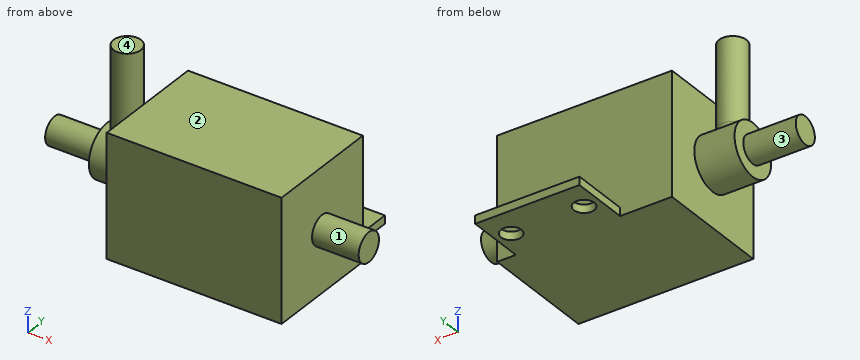
from build123d import *

# Parameters (mm, degrees)
SKETCH1_W                            = 30
SKETCH1_H                            = 20
BOSS_EXTRUDE1_DEPTH                  = 21
SKETCH2_W                            = 17.9
SKETCH2_H                            = 1.4
BOSS_EXTRUDE2_DEPTH                  = 10
SKETCH3_R                            = 2.5
BOSS_EXTRUDE3_DEPTH                  = 8
SKETCH4_R                            = 4.5
BOSS_EXTRUDE4_DEPTH                  = 6.9
SKETCH5_R                            = 2.35
BOSS_EXTRUDE5_DEPTH                  = 9
SKETCH7_R                            = 2.35
BOSS_EXTRUDE6_DEPTH                  = 14.2
BOSS_EXTRUDE6_DIRECTION_2_REACH      = 53.391
BOSS_EXTRUDE6_DIRECTION_2_END_RADIUS = 4.5
SKETCH8_2_R                          = 1.75
CUT_EXTRUDE1_DEPTH                   = 56.828666472
SKETCH8_R                            = 1.75
BOSS_EXTRUDE7_DEPTH                  = 27.8


with BuildPart() as part:
    # Sketch1 → Boss-Extrude1 (new body)
    with BuildSketch(Plane.XY):
        with Locations((15, 10)):
            Rectangle(SKETCH1_W, SKETCH1_H)
    extrude(amount=BOSS_EXTRUDE1_DEPTH)

    # Sketch2 → Boss-Extrude2 (add)
    with BuildSketch(Plane(origin=(0, 20, 0), x_dir=(1, 0, 0), z_dir=(0, 1, 0))):
        with Locations((17.85, -0.7)):
            Rectangle(SKETCH2_W, SKETCH2_H)
    extrude(amount=BOSS_EXTRUDE2_DEPTH)

    # Sketch3 → Boss-Extrude3 (add)
    with BuildSketch(Plane(origin=(30, 0, 0), x_dir=(0, 0, -1), z_dir=(1, 0, 0))):
        with Locations((-10.5, 10)):
            Circle(SKETCH3_R)
    extrude(amount=BOSS_EXTRUDE3_DEPTH)

    # Sketch4 → Boss-Extrude4 (add)
    with BuildSketch(Plane.ZY):
        with Locations(Location((10.5, 10, 0), (0, 0, 180))):
            Circle(SKETCH4_R)
    extrude(amount=BOSS_EXTRUDE4_DEPTH)

    # Sketch5 → Boss-Extrude5 (add)
    with BuildSketch(Plane.ZY.offset(6.9)):
        with Locations((10.5, 10)):
            Circle(SKETCH5_R)
    extrude(amount=BOSS_EXTRUDE5_DEPTH)

    # Sketch7 → Boss-Extrude6 (add)
    with BuildSketch(Plane(origin=(-6.9, 10, 15), x_dir=(1, 0, 0), z_dir=(0, 0, 1))):
        with Locations((3.45, 0)):
            Circle(SKETCH7_R)
    extrude(amount=BOSS_EXTRUDE6_DEPTH)

    # Boss-Extrude6 direction 2: up to this cylinder (the profile starts outside it)
    boss_extrude6_direction_2_end = Plane(origin=(-3.45, 10, 10.5), z_dir=(1, 0, 0)) * Cylinder(BOSS_EXTRUDE6_DIRECTION_2_END_RADIUS, 116.782, mode=Mode.PRIVATE)
    # Sketch7 → Boss-Extrude6 direction 2 (add, up to the surface)
    with BuildSketch(Plane(origin=(-6.9, 10, 15), x_dir=(1, 0, 0), z_dir=(0, 0, 1)), mode=Mode.PRIVATE) as boss_extrude6_direction_2_sk1:
        with Locations((3.45, 0)):
            Circle(SKETCH7_R)
    boss_extrude6_direction_2_tool1 = extrude(boss_extrude6_direction_2_sk1.sketch, amount=-BOSS_EXTRUDE6_DIRECTION_2_REACH, mode=Mode.PRIVATE) - boss_extrude6_direction_2_end
    add(boss_extrude6_direction_2_tool1.solids().sort_by_distance((-3.45, 10, 15))[0])
    add(boss_extrude6_direction_2_tool1.solids().sort_by_distance((-3.45, 10, 15))[1])

    # Sketch8<2> → Cut-Extrude1 (cut, through all)
    with BuildSketch(Plane.XY.offset(1.4)):
        with Locations((11.6, 25)):
            Circle(SKETCH8_2_R)
        with Locations(Location((24.1, 25, 0), (0, 0, 180))):
            Circle(SKETCH8_2_R)
    extrude(amount=-CUT_EXTRUDE1_DEPTH, mode=Mode.SUBTRACT)

    # Sketch8 → Boss-Extrude7 (add, through all)
    with BuildSketch(Plane.XY.offset(1.4)):
        with Locations((11.6, 25)):
            Circle(SKETCH8_R)
        with Locations(Location((24.1, 25, 0), (0, 0, 180))):
            Circle(SKETCH8_R)
    extrude(amount=BOSS_EXTRUDE7_DEPTH)


with BuildPart() as boss_extrude7_kept_piece:
    # of the separate pieces the step leaves, the one the design keeps (boss_extrude7_pieces_kept)
    add(part.part.solids().sort_by_distance((0, 0, 0))[0])


solid = boss_extrude7_kept_piece.part
Geometry check sheet. Reference: the model listing, model coordinates, mm. Face numbers are marked on the shaded views. A direction names the side the tool comes from. Give positions to 0.01 mm unless a question says otherwise; leave off trailing zeros. Order: outer loops, then holes, each group sorted by start corner. A loop starts at its lowest first (then second) coordinate and runs counter-clockwise, first axis right, second up.
1) Cross-section at B-B (z = 17). Record the boundary of the cut face in (x, y).
Results are:
outline: circle Ø4.7 at (-3.45, 10); (0, 0) - (30, 0) - (30, 20) - (0, 20) - close
2) Cross-section at D-D (z = 10.5). Record the boundary of the cut face in (x, y).
Results are:
outline: (-15.9, 7.65) - (-6.9, 7.65) - (-6.9, 5.5) - (0, 5.5) - (0, 0) - (30, 0) - (30, 7.5) - (38, 7.5) - (38, 12.5) - (30, 12.5) - (30, 20) - (0, 20) - (0, 14.5) - (-6.9, 14.5) - (-6.9, 12.35) - (-15.9, 12.35) - close
3) Material ranges on probe 1 along Y at (x, z) = (11.6, 0.55); probe 2 along X at (y, z) = (15.25, 8); probe 3 along Z at (x, y) = (7, 5), recorded low to high.
Results are:
probe 1: y = 0 to 23.25, 26.75 to 30
probe 2: x = 0 to 30
probe 3: z = 0 to 21
4) Cross-section at A-A (x = 24.1). Record the boundary of the cut face in (y, z), then the cut area to 3 significant figures.
Results are:
outline: (0, 0) - (23.25, 0) - (23.25, 1.4) - (20, 1.4) - (20, 21) - (0, 21) - close; (26.75, 0) - (30, 0) - (30, 1.4) - (26.75, 1.4) - close
area: 429 mm2
5) Cross-section at C-C (y = 24.25). Record the boundary of the cut face in (x, z).
Results are:
outline: (8.9, 0) - (10.02, 0) - (10.02, 1.4) - (8.9, 1.4) - close; (13.18, 0) - (22.52, 0) - (22.52, 1.4) - (13.18, 1.4) - close; (25.68, 0) - (26.8, 0) - (26.8, 1.4) - (25.68, 1.4) - close
6) Tool access check on the marked faces 1, 2, 3 and 4. Record the directions out of +Z, -Z, +X, -X, +Y, -Y that give a thin tool (end or side, any length) a straight path to the whole face; none if there is none.
Results are:
face 1: +X
face 2: +Z, +X, +Y, -Y
face 3: -X
face 4: +Z, +X, -X, +Y, -Y
7) Gauge pin test, flat ends, axial feed: pin 1 (3 mm diameter, centred on x = 26, y = 24, fed in from +Z); pin 2 (6 mm diameter, centred on y = 23, z = 24.5, fed in from +X); pin 3 (6.5 mm diameter, centred on x = 13.5, z = 9.5, fed in from +Y); pin 4 (16 mm diameter, centred on x = 13, y = 7, fed in from +Z). Record the tip position at first contact, or that the pin passes through.
Results are:
pin 1: stops at z = 1.4
pin 2: passes through
pin 3: stops at y = 20
pin 4: stops at z = 21
